Autodesk Inventor part; units mm, degrees
ref_plane "Work Plane1" through (0, -33, 0) normal (0, 1, 0) x (-1, 0, 0)
ref_plane "YZ Plane" through (0, 0, 0) normal (1, 0, 0) x (0, 1, 0)
ref_plane "XY Plane" through (0, 0, 0) normal (0, 0, 1) x (1, 0, 0)
ref_plane "Work Plane1" through (0, -33, 0) normal (0, 1, 0) x (-1, 0, 0)
sketch "Sketch1" plane through (0, -33, 0) normal (0, 1, 0) x (-1, 0, 0)
  line L0 (-65, -10) -> (-65, 10)
  line L1 (16.5, -30) -> (16.5, 10)
  line L2 (16.5, 10) -> (-65, 10)
  line L3 (-10, -30) -> (-65, -10)
  line L4 (16.5, -30) -> (-10, -30)
extrude "Extrusion7" add sketch "Sketch1" along normal blind 61
sketch "Sketch2" plane through (65, -33, 10) normal (1, 0, 0) x (0, 0, -1)
  line L0 (6, 0) -> (40, 0)
  line L1 (40, 55) -> (40, 0)
  line L2 (6, 0) -> (6, 55)
  line L3 (40, 55) -> (6, 55)
extrude "Extrusion6" cut sketch "Sketch2" against normal blind 55
sketch "Sketch3" plane through (65, -33, 10) normal (1, 0, 0) x (0, 0, -1)
  line L0 (0, 33) -> (6, 33)
  line L1 (0, 0) -> (6, 0)
  line L2 (6, 0) -> (6, 33)
  line L3 (0, 0) -> (0, 33)
extrude "Extrusion5" cut sketch "Sketch3" against normal blind 12
sketch "Sketch4" plane through (-16.5, -33, -30) normal (-1, 0, 0) x (0, 0, 1)
  line L0 (0, 0) -> (40, 0)
  line L1 (0, 33) -> (0, 0)
  line L2 (40, 33) -> (0, 33)
  line L3 (40, 0) -> (40, 33)
extrude "Extrusion4" cut sketch "Sketch4" against normal blind 22.5
sketch "Sketch5" plane through (65, 22, 4) normal (0, 0, -1) x (-1, 0, 0)
  line L0 (9.5, 0) -> (2.5, 0)
  line L1 (9.5, 6) -> (2.5, 6)
  line L2 (9.5, 6) -> (9.5, 0)
  line L3 (2.5, 6) -> (2.5, 0)
extrude "Extrusion3" cut sketch "Sketch5" along normal blind 5
sketch "Sketch6" plane through (10, 28, -30) normal (0, 0, -1) x (-1, 0, 0)
  line L0 (10, 0) -> (26.5, 0)
  line L1 (26.5, 0) -> (26.5, -28)
  line L2 (10, -28) -> (26.5, -28)
  line L3 (10, 0) -> (10, -28)
extrude "Extrusion2" cut sketch "Sketch6" against normal blind 30
sketch "Sketch7" plane through (65, 22, -1) normal (0, 0, 1) x (1, 0, 0)
  line L0 (-8.25, 0) -> (-3.75, 0)
  line L1 (-3.75, 6) -> (-3.75, 0)
  line L2 (-8.25, 6) -> (-8.25, 0)
  line L3 (-8.25, 6) -> (-3.75, 6)
extrude "Extrusion1" cut sketch "Sketch7" against normal blind 5 draft 0
chamfer "Chamfer1" distance 34 distance2 33 1 edges at (8, -33, -30) measured on face at (23, -33, 8)
hole "Hole12" at (38, 22, -8) direction (0, 1, 0) diameter 4.5 depth 6
hole "Hole11" at (18, 22, -8) direction (0, 1, 0) diameter 4.5 depth 6
hole "Hole10" at (10, 17.5, -24) direction (-1, 0, 0) diameter 4.5 depth 10
hole "Hole9" at (59, 20, 10) direction (0, 0, -1) diameter 4.5 depth 6
hole "Hole8" at (59, 4, 10) direction (0, 0, -1) diameter 4.5 depth 6
hole "Hole7" at (-10.5, 20, 10) direction (0, 0, -1) diameter 4.5 depth 10
sketch "Sketch13" plane through (-16.5, 28, 10) normal (0, 0, 1) x (1, 0, 0)
  point P0 (6, -8)
hole "Hole6" at (47.5, 3.5, 4) direction (0, 0, 1) diameter 3.5 depth 6
sketch "Sketch12" plane through (-16.5, 28, 10) normal (0, 0, 1) x (1, 0, 0)
  point P0 (75.5, -24)
hole "Hole5" at (47.5, -27.5, 4) direction (0, 0, 1) diameter 3.5 depth 6
sketch "Sketch11" plane through (-16.5, 28, 10) normal (0, 0, 1) x (1, 0, 0)
  point P0 (75.5, -8)
hole "Hole4" at (16.5, -27.5, 4) direction (0, 0, 1) diameter 3.5 depth 6
sketch "Sketch10" plane through (10, -33, 10) normal (1, 0, 0) x (0, 0, -1)
  point P0 (34, 50.5)
hole "Hole3" at (16.5, 3.5, 4) direction (0, 0, 1) diameter 3.5 depth 6
sketch "Sketch9" plane through (65, 22, -10) normal (0, -1, 0) x (1, 0, 0)
  point P0 (-47, 2)
hole "Hole2" at (32, -12, 4) direction (0, 0, 1) diameter 24 depth 6
sketch "Sketch8" plane through (65, 22, -10) normal (0, -1, 0) x (1, 0, 0)
  point P0 (-27, 2)
hole "Hole1" at (-10.5, 4, 10) direction (0, 0, -1) diameter 4.5 depth 10
sketch "Sketch14" plane through (65, 0, 4) normal (0, 0, -1) x (-1, 0, 0)
  point P0 (17.5, 3.5)
sketch "Sketch15" plane through (65, 0, 4) normal (0, 0, -1) x (-1, 0, 0)
  point P0 (17.5, -27.5)
sketch "Sketch16" plane through (65, 0, 4) normal (0, 0, -1) x (-1, 0, 0)
  point P0 (48.5, -27.5)
sketch "Sketch17" plane through (65, 0, 4) normal (0, 0, -1) x (-1, 0, 0)
  point P0 (48.5, 3.5)
sketch "Sketch18" plane through (65, 0, 4) normal (0, 0, -1) x (-1, 0, 0)
  point P0 (33, -12)
sketch "Sketch19" plane through (-16.5, 28, 10) normal (0, 0, 1) x (1, 0, 0)
  point P0 (6, -24)
properties part number "Hopper Motor Holder" material "ASA Plastic"
Check sheet for the modelled part. Datum: model origin and axes. Units: mm. A direction names the side the tool comes from. Coordinates: 2 decimals unless noted, no trailing zeros. Order: outer loops, then holes, each group sorted by start corner. A loop starts at its lowest first (then second) coordinate and runs counter-clockwise, first axis right, second up. Notation, with made-up numbers: (-3.75, -4) -> (7.25, -4) arc R19 ccw to (7.25, 32) -> close; hole circle Ø3 at (-18, -28). An arc over 180 degrees is marked (long way). Write item = value, one per line. Start each with the question number.
1) Access from +Z, -Z, +X, -X, +Y, -Y to the whole of each face (thin tool, end or side, straight path). Record for faces 1 (the flat face through (2, 0, -1)), 2 (the flat face through (-8, 14, 0)), 3 (the flat face through (53, -16, 7)), 4 (the flat face through (62.5, 25, 2)).
2) Go/stop test with flat-tipped pins: P1, Ø8, axis at y = 10, z = -16.5, coming from the -X side; P2, Ø8, axis at x = 34, y = -4, coming from the -Z side; P3, Ø6, axis at x = 49.5, z = -17.5, coming from the +Y side; P4, Ø8, axis at x = 23, z = -9.5, coming from the -Y side. Record where each tip stops, or that it passes through.
3) Cross-section at A-A (x = 32). Enter the section's corners in (y, z), then the cut area to 3 significant figures.
4) Cross-section at D-D (z = -8). Enter the section's corners in (x, y), then the cut area to 3 significant figures.
5) Material ranges on L1, parallel to Y at x = 47.5, z = 5.75; L2, parallel to X at y = 20, z = 6.7; L3, parallel to X at y = 4, z = 6.25, recorded low to high.
6) Cross-section at C-C (y = 4). Enter the section's corners in (x, z), then the cut area to 3 significant figures.
7) Cross-section at B-B (z = 7). State how many separate pieces and enclosed holes the cut face has, then the cut area to 3 significant figures.
8) Mould release check, pull along Y, two halves, no side actions. Record for faces 5 (the flat face through (32, 22, -9)), 6 (the cylindrical face through (23.89, -20.844, 7.042)), 7 (the flat face through (6, -13, -6)): +Y half, -Y half, draft (parallel to the pull), parting line (faces both ways), or undercut.
Ans:
q1.face_1 = +Z, -Z, -X, -Y
q1.face_2 = -Z, -X, +Y, -Y
q1.face_3 = +Z, -Z, +X, -Y
q1.face_4 = +Y, -Y
q2.P1 = 0
q2.P2 = 4
q2.P3 = 28
q2.P4 = 22
q3.outline = (-33, 4) -> (-24, 4) -> (-24, 10) -> (-33, 10) -> close; (0, 4) -> (22, 4) -> (22, -22) -> (28, -22) -> (28, 10) -> (0, 10) -> close
q3.area = 378 mm²
q4.outline = (0, 0) -> (6, 0) -> (6, -21.35) -> (10, -21.35) -> (10, 22) -> (15.75, 22) -> (15.75, 28) -> (0, 28) -> close; (20.25, 22) -> (35.75, 22) -> (35.75, 28) -> (20.25, 28) -> close; (40.25, 22) -> (65, 22) -> (65, 28) -> (40.25, 28) -> close
q4.area = 641 mm²
q5.L1 = -33 to -29.25, -25.75 to 1.75, 5.25 to 28
q5.L2 = -16.5 to -12.75, -8.25 to 56.75, 61.25 to 65
q5.L3 = -16.5 to -12.75, -8.25 to 14.82, 18.18 to 45.82, 49.18 to 56.75, 61.25 to 65
q6.outline = (-16.5, 0) -> (-12.75, 0) -> (-12.75, 10) -> (-16.5, 10) -> close; (-8.25, 0) -> (0, 0) -> (0, -30) -> (10, -30) -> (10, 4) -> (14.82, 4) -> (14.82, 10) -> (-8.25, 10) -> close; (18.18, 4) -> (45.82, 4) -> (45.82, 10) -> (18.18, 10) -> close; (49.18, 4) -> (56.75, 4) -> (56.75, 10) -> (49.18, 10) -> close; (61.25, 4) -> (65, 4) -> (65, 10) -> (61.25, 10) -> close
q6.area = 783 mm²
q7.separate_pieces = 1
q7.enclosed_holes = 9
q7.area = 3,280 mm²
q8.face_5 = -Y half
q8.face_6 = undercut
q8.face_7 = draft
